from build123d import *

# Parameters (mm, degrees)
F0_W     = 6
F0_H     = 66
F1_DEPTH = 2
F3_DEPTH = 2
F5_DEPTH = 5
F6_R     = 1.5
F7_DEPTH = 2
F8_R     = 2.99999


# Not quite as in the source:
# - a fillet or chamfer is up to 0.001 mm smaller than in the source, because OpenCascade refuses the exact size


with BuildPart() as f1:
    # F0 (on Top) → F1 (new body)
    with BuildSketch(Plane.XY):
        Rectangle(F0_W, F0_H)
    extrude(amount=F1_DEPTH)

    # F2 (on face) → F3 (cut, through all)
    with BuildSketch(Plane.XY.offset(2)):
        with BuildLine():
            ThreePointArc((0, -1.5), (1.0606601718, -1.0606601718), (1.5, 0))
            ThreePointArc((1.5, 0), (1.0606601718, 1.0606601718), (0, 1.5))
            Line((0, 1.5), (0, 0))
            Line((0, 0), (0, -1.5))
        make_face()
        with BuildLine():
            ThreePointArc((1.75, -30), (1.2374368671, -28.7625631329), (0, -28.25))
            ThreePointArc((0, -28.25), (-1.2374368671, -31.2374368671), (1.75, -30))
        make_face()
        with BuildLine():
            ThreePointArc((1.75, 30), (-1.2374368671, 31.2374368671), (0, 28.25))
            ThreePointArc((0, 28.25), (1.2374368671, 28.7625631329), (1.75, 30))
        make_face()
        with BuildLine():
            Line((0, 0), (0, 1.5))
            ThreePointArc((0, 1.5), (-1.5, 0), (0, -1.5))
            Line((0, -1.5), (0, 0))
        make_face()
    extrude(amount=-F3_DEPTH, mode=Mode.SUBTRACT)

    # F4 (on face) → F5 (join)
    with BuildSketch(Plane.YZ.offset(3)):
        Polygon((3, 2), (0, 2), (-3, 2), (-3, 0), (0, 0), (3, 0), align=None)
    extrude(amount=F5_DEPTH)

    # F6 (on face) → F7 (cut, through all)
    with BuildSketch(Plane.XY.offset(2)):
        with Locations((5.0139404441, 0)):
            Circle(F6_R)
    extrude(amount=-F7_DEPTH, mode=Mode.SUBTRACT)

    # F8 (radius 3 in the source; OpenCascade refuses exactly that, so slightly less here)
    f8_edges = [f1.edges().sort_by_distance(p)[0] for p in [
        (-3, -33, 1),
        (3, -33, 1),
        (3, 33, 1),
        (-3, 33, 1),
        (8, -3, 1),
        (8, 3, 1),
    ]]
    fillet(f8_edges, radius=F8_R)


solid = f1.part
Geometry: final body of the model. Coordinates: model frame, mm. A direction names the side the tool comes from. Coordinates: 2 decimals unless noted, no trailing zeros. Order: outer loops, then holes, each group sorted by start corner. A loop starts at its lowest first (then second) coordinate and runs counter-clockwise, first axis right, second up.
(1) Draft query along X for faces 1 (the face through (2, 0, 0)), 2 (the face through (-3, 0, 1)), 3 (the face through (6.445, 0.451, 1.014)). Return one class per face: pulls with the +X half, pulls with the -X half, needs draft (parallel to the pull), parting line crosses it, or undercut.
(2) Section query B-B (y = -22.5). Return the cut outline in (x, z).
(3) First-contact query: pin 1 (1 mm diameter, centred on x = -1, z = 0.5, fed in from -Y); pin 2 (1 mm diameter, centred on x = 4, z = 1.5, fed in from +Y). Flat tips, straight axial feed; report the tip coordinate or a pass-through.
(4) Access query for faces 4 (the face through (4, 3, 1)), 5 (the face through (-2.14, 32.1, 1.01)), 6 (the face through (3, -17, 1)). Directions: +Z, -Z, +X, -X, +Y, -Y. A direction counts if a zero-diameter tool reaches every point of the face in a straight line with its end or side. Return the directions, or none.
(5) Section query A-A (z = 0.7). State how many separate pieces and enclosed holes the cut face has, plus the area to 3 significant figures.
(6) Material intervals for probe 1 along X at (y, z) = (-30, 0.85); probe 2 along Y at (x, z) = (0.75, 0.8); probe 3 along X at (y, z) = (-25.5, 1.55), sorted ascending.
Solution:
1. face 1: needs draft
1. face 2: pulls with the -X half
1. face 3: undercut
2. outline: (-3, 0) - (3, 0) - (3, 2) - (-3, 2) - close
3. pin 1: stops at y = -32.96
3. pin 2: stops at y = 3
4. face 4: +Z, -Z, +X, +Y
4. face 5: +Z, -Z, -X, +Y
4. face 6: +Z, -Z, +X, -Y
5. separate pieces: 1
5. enclosed holes: 4
5. area: 381 mm2
6. probe 1: x = -3 to -1.75, 1.75 to 3
6. probe 2: y = -32.9 to -31.58, -28.42 to -1.3, 1.3 to 28.42, 31.58 to 32.9
6. probe 3: x = -3 to 3
